Design review of the part built by this model. Coordinates are the model's own, in mm. A direction names the side the tool comes from. Give positions to 0.01 mm unless a question says otherwise; leave off trailing zeros. Loops run counter-clockwise (first coordinate to the right, second up) from the corner with the lowest first, then second, coordinate; pieces in that order, holes last. Notation, with made-up numbers: (38, 1.25) -> (87, 1.25) arc R29 cw to (87, 38.25) -> close; hole circle Ø8 at (74, -13). An arc over 180 degrees is marked (long way). Use a Markdown table: item, result. Add a question column.
1. Add section A-A (x = -18.5). State the section outline as (y, z) points.
2. Add section C-C (y = -42.5). State the section outline as (x, z) points.
3. Add section D-D (x = 36.5). State the section outline as (y, z) points.
4. To check wall thickness, follow line 1 (Y direction, x = 36.5, z = 0.85); line 2 (Y direction, x = -56, z = 1.6); line 3 (X direction, y = -6, z = 0.25). State the ranges of each line that lie inside material, in increasing order.
5. Draft analysis for pull direction Y (two halves, no side actions). For faces 1 (the flat face through (41.151, 15, 1)), 2 (the flat face through (-1, -52.5, 1)), 3 (the flat face through (1, 40.5, 1)), 4 (the flat face through (-1, 52.5, 1)), state which applies: pulls with the +Y half, pulls with the -Y half, needs draft (parallel to the pull), parting line crosses it, or undercut.
6. Add section B-B (y = 12). State the section outline as (x, z) points.
7. For faces 5 (the flat face through (-40, 15, 1)), 6 (the flat face through (-1, -11, 3)), list the 3-axis set-ups (+Z, -Z, +X, -X, +Y, -Y) from which the entire face can be reached by the end or side of a thin tool; tool diameter is ignored.
8. For pin 1 Ø5 at (x, y) = (-56, -48.5) entering from +Z, flat-tipped, find the tip position at first contact; note if it passes through.
```python
from build123d import *

# Parameters (mm, degrees)
SKETCH_1_W          = 120
SKETCH_1_H          = 105
EXTRUDE_1_DEPTH     = 3
SKETCH_2_R          = 1.5
CUT_EXTRUDE_1_DEPTH = 10
SKETCH_3_R          = 1.5
SKETCH_3_W          = 81.151446905
SKETCH_3_H          = 50
CUT_EXTRUDE_2_DEPTH = 10


with BuildPart() as part:
    # 草图1 → 凸台-拉伸1 (new body)
    with BuildSketch(Plane.XY):
        Rectangle(SKETCH_1_W, SKETCH_1_H)
    extrude(amount=EXTRUDE_1_DEPTH)

    # 草图2 → 切除-拉伸1 (cut)
    with BuildSketch(Plane.XY.offset(3)):
        with Locations((-56, 48.5)):
            Circle(SKETCH_2_R)
        with Locations((56, 48.5)):
            Circle(SKETCH_2_R)
        with Locations((56, -48.5)):
            Circle(SKETCH_2_R)
        with Locations((-56, -48.5)):
            Circle(SKETCH_2_R)
    extrude(amount=-CUT_EXTRUDE_1_DEPTH, mode=Mode.SUBTRACT)

    # 草图3 → 切除-拉伸2 (cut)
    with BuildSketch(Plane(origin=(0, 0, 0), x_dir=(-1, 0, 0), z_dir=(0, 0, -1))):
        with Locations((-36.5, -42.5)):
            Circle(SKETCH_3_R)
        with Locations((35.5, -42.5)):
            Circle(SKETCH_3_R)
        with Locations((-36.5, -16.5)):
            Circle(SKETCH_3_R)
        with Locations((35.5, -16.5)):
            Circle(SKETCH_3_R)
        with Locations((-0.575723453, 15.5)):
            Rectangle(SKETCH_3_W, SKETCH_3_H)
    extrude(amount=-CUT_EXTRUDE_2_DEPTH, mode=Mode.SUBTRACT)


solid = part.part
```
Taken from the geometry:
| question | item | result |
|---|---|---|
| 1 | outline | (-52.5, 0) -> (-9.5, 0) -> (-9.5, 3) -> (-52.5, 3) -> close; (40.5, 0) -> (52.5, 0) -> (52.5, 3) -> (40.5, 3) -> close |
| 2 | outline | (-60, 0) -> (-37, 0) -> (-37, 3) -> (-60, 3) -> close; (-34, 0) -> (35, 0) -> (35, 3) -> (-34, 3) -> close; (38, 0) -> (60, 0) -> (60, 3) -> (38, 3) -> close |
| 3 | outline | (-52.5, 0) -> (-44, 0) -> (-44, 3) -> (-52.5, 3) -> close; (-41, 0) -> (-18, 0) -> (-18, 3) -> (-41, 3) -> close; (-15, 0) -> (-9.5, 0) -> (-9.5, 3) -> (-15, 3) -> close; (40.5, 0) -> (52.5, 0) -> (52.5, 3) -> (40.5, 3) -> close |
| 4 | line 1 | y = -52.5 to -44, -41 to -18, -15 to -9.5, 40.5 to 52.5 |
| 4 | line 2 | y = -52.5 to -50, -47 to 47, 50 to 52.5 |
| 4 | line 3 | x = -60 to -40, 41.15 to 60 |
| 5 | face 1 | undercut |
| 5 | face 2 | pulls with the -Y half |
| 5 | face 3 | undercut |
| 5 | face 4 | pulls with the +Y half |
| 6 | outline | (-60, 0) -> (-40, 0) -> (-40, 3) -> (-60, 3) -> close; (41.15, 0) -> (60, 0) -> (60, 3) -> (41.15, 3) -> close |
| 7 | face 5 | +Z, -Z |
| 7 | face 6 | +Z, +X, -X, +Y, -Y |
| 8 | pin 1 | stops at z = 3 |
